For this review, take the finished solid that the model builds, in its own axes (mm). Face numbers are marked on the shaded views. A direction names the side the tool comes from. Round coordinates to 2 decimals unless told otherwise and drop trailing zeros. Order: outer loops, then holes, each group sorted by start corner. A loop starts at its lowest first (then second) coordinate and runs counter-clockwise, first axis right, second up. Notation, with made-up numbers: M 60.5,7.5 L 80.5,7.5 A8 cw 80.5,15.5 Z; hole C -13,21.25 d8. An arc over 180 degrees is marked long. Use a Markdown table: item, result.
Autodesk Inventor part; units mm, degrees
ref_plane "YZ Plane" through (0, 0, 0) normal (1, 0, 0) x (0, 1, 0)
ref_plane "XZ Plane" through (0, 0, 0) normal (0, 1, 0) x (-1, 0, 0)
ref_plane "XY Plane" through (0, 0, 0) normal (0, 0, 1) x (1, 0, 0)
sketch "Sketch1" plane through (0, 0, 0) normal (0, 1, 0) x (-1, 0, 0)
  line L0 (98.425, 38.1) -> (-98.425, 38.1)
  line L1 (-98.425, 38.1) -> (-98.425, -38.1)
  line L2 (-98.425, -38.1) -> (98.425, -38.1)
  line L3 (98.425, -38.1) -> (98.425, 38.1)
  line L4 (98.425, 38.1) -> (-98.425, -38.1) construction
  line L5 (-98.425, 38.1) -> (98.425, -38.1) construction
  point P0 (0, 0)
  dimension "length" = 196.85
  dimension "width" = 76.2
extrude "Extrusion1" add sketch "Sketch1" along normal blind 19.05
sketch "Sketch3" plane through (0, 19.05, 0) normal (0, 1, 0) x (1, 0, 0)
  line L0 (98.425, 38.1) -> (-98.425, 38.1)
  line L1 (-98.425, 38.1) -> (98.425, 38.1)
  line L2 (98.425, 38.1) -> (98.425, 0)
  line L3 (98.425, -38.1) -> (98.425, 38.1)
  line L4 (98.425, 0) -> (85.725, 0)
  line L5 (85.725, 0) -> (85.725, 25.4)
  line L6 (85.725, 25.4) -> (-85.725, 25.4)
  line L7 (-85.725, 25.4) -> (-85.725, 0)
  line L8 (-85.725, 0) -> (-98.425, 0)
  line L9 (-98.425, 38.1) -> (-98.425, -38.1)
  line L10 (-98.425, 0) -> (-98.425, 38.1)
  point P0 (0, 0)
  dimension "d9" = 38.1
  dimension "batterSupportSideEdge" = 12.7
  dimension "batterySupportCutOut" = 25.4
  dimension "d28" = 12.7
extrude "Extrusion2" add sketch "Sketch3" along normal blind 25.4
sketch "Sketch4" plane through (0, 44.45, 0) normal (0, 1, 0) x (1, 0, 0)
  line L0 (98.425, 38.1) -> (-98.425, 38.1) construction
  line L1 (0, 38.1) -> (0, 25.4) construction
  line L2 (-85.725, 25.4) -> (85.725, 25.4)
  point P0 (0, 0)
  point P1 (0, 31.75)
  dimension "d14" = 6.35
hole "Hole1" at (0, 44.45, -31.75) direction (0, -1, 0) diameter 10.0838 end through all
sketch "Sketch5" plane through (0, 19.05, 0) normal (0, 1, 0) x (1, 0, 0)
  line L0 (-60.325, -38.1) -> (60.325, -38.1)
  line L1 (60.325, -38.1) -> (60.325, 0)
  line L2 (60.325, 0) -> (-60.325, 0)
  line L3 (-60.325, 0) -> (-60.325, -38.1)
  line L4 (-98.425, 0) -> (-98.425, -38.1)
  line L5 (98.425, -38.1) -> (98.425, 0)
  line L6 (85.725, 25.4) -> (-85.725, 25.4)
  point P0 (0, 0)
  dimension "d22" = 38.1
  dimension "d23" = 38.1
  dimension "d24" = 25.4
extrude "Extrusion3" cut sketch "Sketch5" against normal through all
properties part number "BatteryHolder"
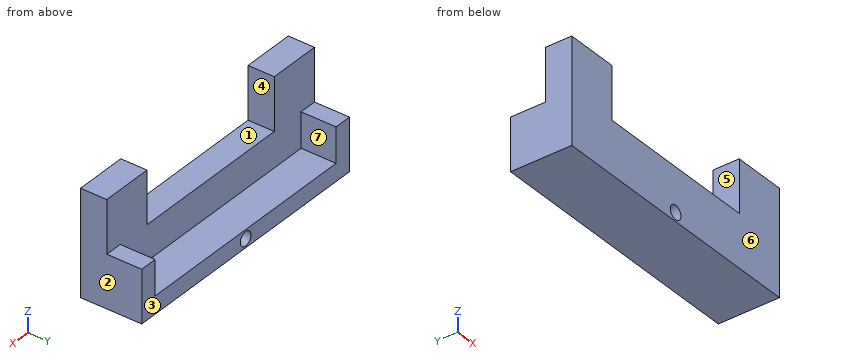
Q1. Clearance check with flat-ended pins moving along their axes: pin 1 (1.5 mm diameter, centred on x = -70.5, y = 23.5, fed in from +Z); pin 2 (19 mm diameter, centred on x = -28.5, z = 0, fed in from +Y); pin 3 (10 mm diameter, centred on x = 93.5, y = 33.5, fed in from +Z). State where each tip first meets the part, or that it passes through.
Determined:
| item | result |
|---|---|
| pin 1 | stops at z = -25.4 |
| pin 2 | stops at y = 19.05 |
| pin 3 | stops at z = 0 |
Q2. Wall thickness on line 1 along X through (y, z) = (42, -1) (3 decimals); line 2 along Z through (x, y) = (0, 25); line 3 along X through (y, z) = (27, -31.75) (3 decimals): over which ranges is each line inside the solid? List them lowest first. Write a range as [from, to].
Determined:
| item | result |
|---|---|
| line 1 | x = [-98.425, -85.725], [85.725, 98.425] |
| line 2 | z = [-38.1, -36.79], [-26.71, -25.4] |
| line 3 | x = [-98.425, -5.042], [5.042, 98.425] |
Q3. Machinability: for the marked faces 5, 6 and 7, which of the approach directions +Z, -Z, +X, -X, +Y, -Y give a long, thin tool a straight path to every point of the face, cutting with its end or side? Answer none if there is none.
Determined:
| item | result |
|---|---|
| face 5 | +Z, +Y, -Y |
| face 6 | +Z, -Z, +X, -X, -Y |
| face 7 | +Z, +Y |
Q4. Add section A-A (z = 15). Write out the cut boundary in (x, y) (3 decimals).
Determined:
| item | result |
|---|---|
| outline | M -98.425,0 L -60.325,0 L -60.325,19.05 L -98.425,19.05 Z; M 60.325,0 L 98.425,0 L 98.425,19.05 L 60.325,19.05 Z |
Q5. Add section B-B (x = 0). Write out the cut boundary in (y, z).
Determined:
| item | result |
|---|---|
| outline | M 0,-38.1 L 44.45,-38.1 L 44.45,-36.79 L 0,-36.79 Z; M 0,-26.71 L 44.45,-26.71 L 44.45,-25.4 L 19.05,-25.4 L 19.05,0 L 0,0 Z |
Q6. Add section D-D (z = -14). Write out the cut boundary in (x, y) (3 decimals), then the cut area to 3 significant figures.
Determined:
| item | result |
|---|---|
| outline | M -98.425,0 L 98.425,0 L 98.425,44.45 L 85.725,44.45 L 85.725,19.05 L -85.725,19.05 L -85.725,44.45 L -98.425,44.45 Z |
| area | 4,400 mm^2 |
Q7. Add section C-C (y = 14). Write out the cut boundary in (x, z) (3 decimals), then the cut area to 3 significant figures.
Determined:
| item | result |
|---|---|
| outline | M -98.425,-38.1 L 98.425,-38.1 L 98.425,38.1 L 60.325,38.1 L 60.325,0 L -60.325,0 L -60.325,38.1 L -98.425,38.1 Z; hole C 0,-31.75 d10.084 |
| area | 10,300 mm^2 |
Q8. Draft analysis for pull direction X (two halves, no side actions). For the marked faces 1, 2, 3 and 4, state which applies: pulls with the +X half, pulls with the -X half, needs draft (parallel to the pull), parting line crosses it, or undercut.
Determined:
| item | result |
|---|---|
| face 1 | undercut |
| face 2 | pulls with the +X half |
| face 3 | needs draft |
| face 4 | undercut |
